Part model, mm, in its own coordinate system. Face numbers are marked on the shaded views. A direction names the side the tool comes from. Round coordinates to 2 decimals unless told otherwise and drop trailing zeros. Order: outer loops, then holes, each group sorted by start corner. A loop starts at its lowest first (then second) coordinate and runs counter-clockwise, first axis right, second up. Notation, with made-up numbers: (7.25, 17.25) - (20.25, 17.25) arc R7 cw to (20.25, 22.25) - close; hole circle Ø2 at (-10.75, 82.25). An arc over 180 degrees is marked (long way). Return JSON: item names as keys, results as strings. Group by question number.
Item 1: Tool access for the marked faces 5 and 6: list every direction of +Z, -Z, +X, -X, +Y, -Y with a clear straight run to the whole face (end or side of a thin tool).
Item 2: Saw through at A-A on z = -18. List the corners of the cut face in (x, y).
Item 3: Probe probe 1 along Z at (x, y) = (74, 37); probe 2 along Y at (x, z) = (104, -31); probe 3 along Z at (x, y) = (76, 18.5). List the from-to ranges inside material, lowest first.
Item 4: Two-plate mould, pull along Y, no slides. Class the marked faces 1, 2, 3 and 4: released by +Y, released by -Y, zero draft, split by the parting line, or undercut.
Item 5: Saw through at B-B on z = -38. List the corners of the cut face in (x, y), and give its area (3 significant figures).
Item 6: Drop flat-ended pins along their axis: pin 1 (6.5 mm diameter, centred on x = 175.62, y = 8.56, fed in from -Z); pin 2 (9 mm diameter, centred on y = 16.39, z = -46.7, fed in from +X); pin 3 (13.5 mm diameter, centred on y = 32.56, z = -40, fed in from -X); pin 4 (3 mm diameter, centred on y = -9.5, z = -18, fed in from +X). Give the stop position or say it passes through.
Item 7: Saw through at D-D on y = 0.5. List the corners of the cut face in (x, z), and give its area (3 significant figures).
Item 8: Saw through at C-C on x = 102. List the corners of the cut face in (y, z), and give its area (3 significant figures).
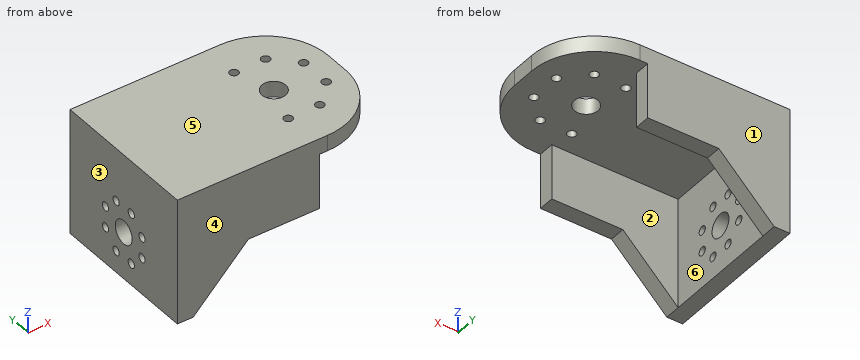
```python
from build123d import *

# Parameters (mm, degrees)
SKETCH3_R           = 7.5
SKETCH3_R_2         = 2.75
BOSS_EXTRUDE1_DEPTH = 10
SKETCH4_W           = 10
SKETCH4_H           = 95
BOSS_EXTRUDE2_DEPTH = 70
SKETCH5_W           = 80
SKETCH5_H           = 10
BOSS_EXTRUDE3_DEPTH = 35
SKETCH8_R           = 7.5
SKETCH8_R_2         = 2.75
CUT_EXTRUDE2_DEPTH  = 43.8
CHAMFER1_SIZE       = 35


with BuildPart() as part:
    # Sketch3 → Boss-Extrude1 (new body)
    with BuildSketch(Plane.XY):
        with BuildLine():
            Line((68.617133813, 80.05993294), (163.617133813, 80.05993294))
            ThreePointArc((163.617133813, 80.05993294), (191.90140506, 68.344204188), (203.617133813, 40.05993294))
            Line((203.617133813, 40.05993294), (203.617133813, 25.05993294))
            ThreePointArc((203.617133813, 25.05993294), (191.90140506, -3.224338307), (163.617133813, -14.94006706))
            Line((163.617133813, -14.94006706), (68.617133813, -14.94006706))
            Line((68.617133813, -14.94006706), (68.617133813, 80.05993294))
        make_face()
        with Locations((163.617133813, 32.55993294)):
            Circle(SKETCH3_R, mode=Mode.SUBTRACT)
        with Locations((189.617133813, 42.55993294)):
            Circle(SKETCH3_R_2, mode=Mode.SUBTRACT)
        with Locations((155.617133813, 56.55993294)):
            Circle(SKETCH3_R_2, mode=Mode.SUBTRACT)
        with Locations((175.617133813, 56.55993294)):
            Circle(SKETCH3_R_2, mode=Mode.SUBTRACT)
        with Locations((155.617133813, 8.55993294)):
            Circle(SKETCH3_R_2, mode=Mode.SUBTRACT)
        with Locations((175.617133813, 8.55993294)):
            Circle(SKETCH3_R_2, mode=Mode.SUBTRACT)
        with Locations((189.617133813, 22.55993294)):
            Circle(SKETCH3_R_2, mode=Mode.SUBTRACT)
    extrude(amount=BOSS_EXTRUDE1_DEPTH)

    # Sketch4 → Boss-Extrude2 (add)
    with BuildSketch(Plane(origin=(0, 0, 0), x_dir=(-1, 0, 0), z_dir=(0, 0, -1))):
        with Locations((-73.617133813, 32.55993294)):
            Rectangle(SKETCH4_W, SKETCH4_H)
    extrude(amount=BOSS_EXTRUDE2_DEPTH)

    # Sketch5 → Boss-Extrude3 (add)
    with BuildSketch(Plane(origin=(0, 0, 0), x_dir=(-1, 0, 0), z_dir=(0, 0, -1))):
        with Locations((-118.617133813, 75.05993294)):
            Rectangle(SKETCH5_W, SKETCH5_H)
        with Locations((-118.617133813, -9.94006706)):
            Rectangle(SKETCH5_W, SKETCH5_H)
    extrude(amount=BOSS_EXTRUDE3_DEPTH)

    # Sketch8 → Cut-Extrude2 (cut)
    with BuildSketch(Plane.ZY.offset(-68.617133813)):
        with Locations(Location((-40, 32.55993294, 0), (0, 0, 270))):
            Circle(SKETCH8_R)
        with Locations(Location((-56.167891819, 25.862972874, 0), (0, 0, 270))):
            Circle(SKETCH8_R_2)
        with Locations(Location((-56.167891819, 39.256893006, 0), (0, 0, 270))):
            Circle(SKETCH8_R_2)
        with Locations(Location((-46.696960066, 48.727824759, 0), (0, 0, 270))):
            Circle(SKETCH8_R_2)
        with Locations(Location((-33.303039934, 48.727824759, 0), (0, 0, 270))):
            Circle(SKETCH8_R_2)
        with Locations(Location((-23.832108181, 39.256893006, 0), (0, 0, 270))):
            Circle(SKETCH8_R_2)
        with Locations(Location((-23.832108181, 25.862972874, 0), (0, 0, 270))):
            Circle(SKETCH8_R_2)
        with Locations(Location((-33.303039934, 16.392041121, 0), (0, 0, 270))):
            Circle(SKETCH8_R_2)
        with Locations(Location((-46.696960066, 16.392041121, 0), (0, 0, 270))):
            Circle(SKETCH8_R_2)
    extrude(amount=-CUT_EXTRUDE2_DEPTH, mode=Mode.SUBTRACT)

    # Chamfer1
    chamfer1_edges = [part.edges().sort_by_distance(p)[0] for p in [
        (78.617133813, 75.05993294, -35),
        (78.617133813, -9.94006706, -35),
    ]]
    chamfer(chamfer1_edges, length=CHAMFER1_SIZE - 0.0001)  # a hair under: the kernel refuses the full size


solid = part.part
```
Filled in:
{
 "1": {"face 5": "+Z, +X, -X, +Y, -Y", "face 6": "-Z, +X"},
 "2": {"outline": "(68.62, -14.94) - (158.62, -14.94) - (158.62, -4.94) - (78.62, -4.94) - (78.62, 70.06) - (158.62, 70.06) - (158.62, 80.06) - (68.62, 80.06) - close"},
 "3": {"probe 1": "z = -70 to -57.74, -54.6 to -46.04, -33.96 to -25.4, -22.26 to 10", "probe 2": "y = -14.94 to -4.94, 70.06 to 80.06", "probe 3": "z = -70 to -48.46, -44.93 to -35.07, -31.54 to 10"},
 "4": {"face 1": "released by +Y", "face 2": "undercut", "face 3": "zero draft", "face 4": "released by -Y"},
 "5": {"outline": "(68.62, -14.94) - (110.62, -14.94) - (110.62, -4.94) - (78.62, -4.94) - (78.62, 25.33) - (68.62, 25.33) - close; (68.62, 39.79) - (78.62, 39.79) - (78.62, 70.06) - (110.62, 70.06) - (110.62, 80.06) - (68.62, 80.06) - close", "area": "1,450 mm^2"},
 "6": {"pin 1": "stops at z = 0", "pin 2": "stops at x = 78.62", "pin 3": "passes through", "pin 4": "stops at x = 158.62"},
 "7": {"outline": "(68.62, -70) - (78.62, -70) - (78.62, 0) - (195.19, 0) - (195.19, 10) - (68.62, 10) - close", "area": "1,970 mm^2"},
 "8": {"outline": "(-14.94, -46.62) - (-4.94, -46.62) - (-4.94, 0) - (70.06, 0) - (70.06, -46.62) - (80.06, -46.62) - (80.06, 10) - (-14.94, 10) - close", "area": "1,880 mm^2"}
}
